Check sheet for the drawn part. Datum: minimum x, y, z corner. Units: mm. A direction names the side the tool comes from. Give positions to 0.01 mm unless a question says otherwise; leave off trailing zeros. Order: outer loops, then holes, each group sorted by start corner. A loop starts at its lowest first (then second) coordinate and runs counter-clockwise, first axis right, second up. Notation, with made-up numbers: (36.25, 44) -> (54.25, 44) arc R23 ccw to (54.25, 57) -> close; hole circle Ø10 at (70.5, -33.5). An arc over 180 degrees is marked (long way). Answer in a Markdown table with one row per item. Add a question column.
(1) Thickness scan on L1, parallel to Y at x = 6.35, z = 1.5; L2, parallel to Y at x = 6, z = 1; L3, parallel to Z at x = 75, y = 2 (1 decimal). Record the ranges inside material, lowest first. Write a range as [from, to].
(2) Cross-section at B-B (z = 14.5). State how many separate pieces and enclosed holes the cut face has, then the cut area to 3 significant figures.
(3) Cross-section at A-A (x = 31.75). Record the cut outline in (y, z).
(4) Cross-section at C-C (x = 139.7). Record the cut outline in (y, z) (1 decimal).
(5) Set-up check for the marked faces 1, 2 and 3: record each of +Z, -Z, +X, -X, +Y, -Y from which the full face is reachable in a straight line by a thin tool's end or side.
(6) Go/stop test with flat-tipped pins: pin 1 (2.5 mm diameter, centred on x = 6.35, y = 34.925, fed in from -Z); pin 2 (10 mm diameter, centred on y = 10.5, z = 22.5, fed in from +X) (1 decimal); pin 3 (8 mm diameter, centred on y = 29, z = 31.5, fed in from +X); pin 4 (8 mm diameter, centred on y = 28.5, z = 25.5, fed in from -X). Record where each tip stops, or that it passes through.
(7) Cross-section at D-D (x = 6.35). Record the cut outline in (y, z) (1 decimal), then the cut area to 3 significant figures.
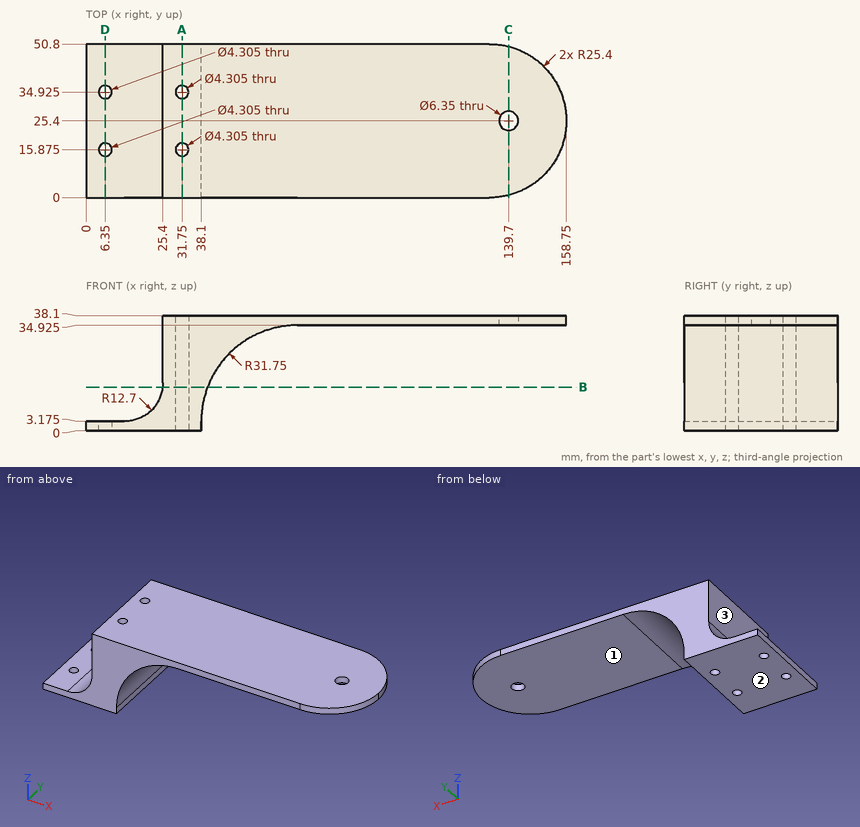
Answer below:
| question | item | result |
|---|---|---|
| 1 | L1 | y = [0, 13.72], [18.03, 32.77], [37.08, 50.8] |
| 1 | L2 | y = [0, 13.75], [18, 32.8], [37.05, 50.8] |
| 1 | L3 | z = [34.9, 38.1] |
| 2 | separate pieces | 1 |
| 2 | enclosed holes | 2 |
| 2 | area | 726 mm² |
| 3 | outline | (0, 0) -> (13.72, 0) -> (13.72, 38.1) -> (0, 38.1) -> close; (18.03, 0) -> (32.77, 0) -> (32.77, 38.1) -> (18.03, 38.1) -> close; (37.08, 0) -> (50.8, 0) -> (50.8, 38.1) -> (37.08, 38.1) -> close |
| 4 | outline | (0.8, 34.9) -> (22.2, 34.9) -> (22.2, 38.1) -> (0.8, 38.1) -> close; (28.6, 34.9) -> (50, 34.9) -> (50, 38.1) -> (28.6, 38.1) -> close |
| 5 | face 1 | -Z, +X, +Y, -Y |
| 5 | face 2 | -Z, +X, -X, +Y, -Y |
| 5 | face 3 | +Z, -X, +Y, -Y |
| 6 | pin 1 | passes through |
| 6 | pin 2 | stops at x = 49.4 |
| 6 | pin 3 | stops at x = 158.7 |
| 6 | pin 4 | stops at x = 25.4 |
| 7 | outline | (0, 0) -> (13.7, 0) -> (13.7, 3.2) -> (0, 3.2) -> close; (18, 0) -> (32.8, 0) -> (32.8, 3.2) -> (18, 3.2) -> close; (37.1, 0) -> (50.8, 0) -> (50.8, 3.2) -> (37.1, 3.2) -> close |
| 7 | area | 134 mm² |
